The listing builds one solid part. Answer for the finished solid, in the listing's coordinates (mm). A direction names the side the tool comes from. Round coordinates to 2 decimals unless told otherwise and drop trailing zeros. Write each loop counter-clockwise with the first axis right and the second up, starting at its lowest first coordinate (ties: lowest second). Pieces come first, ordered by that corner, then holes.
from build123d import *

# Parameters (mm, degrees)
SKETCH1_W            = 130
SKETCH1_H            = 60
BOSS_EXTRUDE1_DEPTH  = 16
CUT_EXTRUDE1_DEPTH   = 135.372616258
SKETCH3_W            = 18.25
SKETCH3_H            = 5.5
CUT_EXTRUDE2_DEPTH   = 2
BOSS_EXTRUDE2_START  = -2
SKETCH3_7_W          = 0.6
SKETCH3_7_H          = 4.9
SKETCH3_7_H_2        = 3.5
BOSS_EXTRUDE2_DEPTH  = 1
SKETCH3_9_W          = 5.875
SKETCH3_9_H          = 3.5
SKETCH3_9_W_2        = 0.6
SKETCH3_9_H_2        = 4.9
SKETCH3_9_W_3        = 17.05
SKETCH3_9_H_3        = 0.6
BOSS_EXTRUDE3_DEPTH  = 2
SKETCH3_10_W         = 5.875
SKETCH3_10_H         = 3.5
BOSS_EXTRUDE4_DEPTH  = 2
SKETCH4_W            = 25
SKETCH4_H            = 8.5
SKETCH4_H_2          = 6.5
CUT_EXTRUDE3_DEPTH   = 128
BOSS_EXTRUDE10_DEPTH = 100
CHAMFER1_SIZE        = 0.8
CHAMFER2_SIZE        = 2


with BuildPart() as part:
    # Sketch1 → Boss-Extrude1 (new body)
    with BuildSketch(Plane(origin=(0, 0, 0), x_dir=(1, 0, 0), z_dir=(0, 1, 0))):
        Rectangle(SKETCH1_W, SKETCH1_H)
    extrude(amount=BOSS_EXTRUDE1_DEPTH)

    # Sketch2 → Cut-Extrude1 (cut, through all)
    with BuildSketch(Plane(origin=(65, 0, 0), x_dir=(0, 0, -1), z_dir=(1, 0, 0))):
        with BuildLine():
            ThreePointArc((-27.5, 16), (-15, 3.5), (-2.5, 16))
            Line((-2.5, 16), (-27.5, 16))
        make_face()
        with BuildLine():
            Line((-27.5, 16), (-2.5, 16))
            ThreePointArc((-2.5, 16), (-15, 28.5), (-27.5, 16))
        make_face()
    extrude(amount=-CUT_EXTRUDE1_DEPTH, mode=Mode.SUBTRACT)

    # Sketch3 → Cut-Extrude2 (cut)
    with BuildSketch(Plane(origin=(65, 0, 0), x_dir=(0, 0, -1), z_dir=(1, 0, 0))):
        with Locations((15, 13.25)):
            Rectangle(SKETCH3_W, SKETCH3_H)
    extrude(amount=-CUT_EXTRUDE2_DEPTH, mode=Mode.SUBTRACT)

    # Sketch3<7> → Boss-Extrude2 (add)
    with BuildSketch(Plane(origin=(65, 0, 0), x_dir=(0, 0, -1), z_dir=(1, 0, 0)).offset(BOSS_EXTRUDE2_START)):
        with Locations((23.825, 13.55)):
            Rectangle(SKETCH3_7_W, SKETCH3_7_H)
        with Locations((23.825, 17.75)):
            Rectangle(SKETCH3_7_W, SKETCH3_7_H_2)
        with Locations((6.175, 17.75)):
            Rectangle(SKETCH3_7_W, SKETCH3_7_H_2)
        with Locations((6.175, 13.55)):
            Rectangle(SKETCH3_7_W, SKETCH3_7_H)
    extrude(amount=BOSS_EXTRUDE2_DEPTH)

    # Sketch3<9> → Boss-Extrude3 (add)
    with BuildSketch(Plane(origin=(65, 0, 0), x_dir=(0, 0, -1), z_dir=(1, 0, 0))):
        with Locations((2.9375, 17.75)):
            Rectangle(SKETCH3_9_W, SKETCH3_9_H)
        Polygon((0, 0), (30, 0), (30, 16), (24.125, 16), (24.125, 11.1), (24.125, 10.5), (23.525, 10.5), (6.475, 10.5), (5.875, 10.5), (5.875, 11.1), (5.875, 16), (0, 16), align=None)
        with Locations((6.175, 13.55)):
            Rectangle(SKETCH3_9_W_2, SKETCH3_9_H_2)
        with Locations((15, 13.55)):
            Rectangle(SKETCH3_9_W_3, SKETCH3_9_H_2)
        with Locations((6.175, 17.75)):
            Rectangle(SKETCH3_9_W_2, SKETCH3_9_H)
        with Locations((15, 17.75)):
            Rectangle(SKETCH3_9_W_3, SKETCH3_9_H)
        with Locations((15, 10.8)):
            Rectangle(SKETCH3_9_W_3, SKETCH3_9_H_3)
        with Locations((6.175, 10.8)):
            Rectangle(SKETCH3_9_W_2, SKETCH3_9_H_3)
        with Locations((23.825, 13.55)):
            Rectangle(SKETCH3_9_W_2, SKETCH3_9_H_2)
        with Locations((23.825, 10.8)):
            Rectangle(SKETCH3_9_W_2, SKETCH3_9_H_3)
        with Locations((23.825, 17.75)):
            Rectangle(SKETCH3_9_W_2, SKETCH3_9_H)
        with Locations((27.0625, 17.75)):
            Rectangle(SKETCH3_9_W, SKETCH3_9_H)
    extrude(amount=BOSS_EXTRUDE3_DEPTH)

    # Sketch3<10> → Boss-Extrude4 (add)
    with BuildSketch(Plane(origin=(65, 0, 0), x_dir=(0, 0, -1), z_dir=(1, 0, 0))):
        with Locations((2.9375, 17.75)):
            Rectangle(SKETCH3_10_W, SKETCH3_10_H)
        with Locations((27.0625, 17.75)):
            Rectangle(SKETCH3_10_W, SKETCH3_10_H)
    extrude(amount=-BOSS_EXTRUDE4_DEPTH)

    # Sketch4 → Cut-Extrude3 (cut)
    with BuildSketch(Plane.ZY.offset(65)):
        with Locations((-15, 11.75)):
            Rectangle(SKETCH4_W, SKETCH4_H)
        with Locations((-15, 19.25)):
            Rectangle(SKETCH4_W, SKETCH4_H_2)
    extrude(amount=-CUT_EXTRUDE3_DEPTH, mode=Mode.SUBTRACT)

    # Sketch5 → Boss-Extrude10 (add)
    with BuildSketch(Plane.ZY.offset(65)):
        Polygon((1.5, 14), (1.5, 11.5), (-1.5, 11.5), (-1.5, 14), (-5, 14), (-5, 0), (5, 0), (5, 14), align=None)
    extrude(amount=BOSS_EXTRUDE10_DEPTH)

    # Chamfer1
    chamfer1_edges = [part.edges().sort_by_distance(p)[0] for p in [
        (-115, 14, -1.5),
        (-115, 14, 1.5),
    ]]
    chamfer(chamfer1_edges, length=CHAMFER1_SIZE)

    # Chamfer2
    chamfer2_edges = [part.edges().sort_by_distance(p)[0] for p in [
        (-65, 16, -28.75),
        (-65, 16, 28.75),
        (-65, 16, 0),
    ]]
    chamfer(chamfer2_edges, length=CHAMFER2_SIZE - 0.0001)  # a hair under: the kernel refuses the full size


solid = part.part
1. Section A-A on x = -123 is taken. Determine the outline of the cut face in (y, z).
Geometry says:
outline: (0, -5) - (14, -5) - (14, -2.3) - (13.2, -1.5) - (11.5, -1.5) - (11.5, 1.5) - (13.2, 1.5) - (14, 2.3) - (14, 5) - (0, 5) - close
2. Section C-C on x = -43.5 is taken. Determine the outline of the cut face in (y, z), plus the area to 3 significant figures.
Geometry says:
outline: (0, -30) - (16, -30) - (16, -27.5) - (7.5, -27.5) - (7.5, -2.5) - (16, -2.5) - (16, 2.5) arc R12.5 cw to (16, 27.5) - (16, 30) - (0, 30) - close
area: 502 mm2
3. A tool of negligible diameter and unlimited length cuts with its end or side. For faces 4 (the face through (63, 10, -15)), 5 (the face through (-114, 7, -5)), 6 (the face through (65, 3, 15)), 7 (the face through (-2, 12, -27.5)), 8 (the face through (-65, 4, 20)), from which of +Z, -Z, +X, -X, +Y, -Y can it reach the whole face along a straight path? Write none if from no direction.
Geometry says:
face 4: +Y
face 5: -Z, -X, +Y, -Y
face 6: +Z, +X, +Y, -Y
face 7: -X, +Y
face 8: +Z, -X, +Y, -Y
4. Given pin 1 (7 mm diameter, centred on y = 5, z = -21, fed in from -X); pin 2 (11 mm diameter, centred on x = -133, y = 8, fed in from +Z); pin 3 (3 mm diameter, centred on x = -13, z = 29, fed in from +Y), each flat-ended and moving along its own axis, determine where each tip first touches the part or whether it passes through.
Geometry says:
pin 1: stops at x = -65
pin 2: stops at z = 5
pin 3: stops at y = 16
5. Section B-B on z = 15 is taken. Determine the outline of the cut face in (x, y), plus the area to 3 significant figures.
Geometry says:
outline: (-65, 0) - (65, 0) - (65, 3.5) - (-65, 3.5) - close
area: 455 mm2
6. For a pull along X with two mould halves and no side action, classify faces 1 (the face through (0.91, 3.503, 15.275)), 2 (the face through (-65, 4, -17)), 3 (the face through (-2, 12, -2.5)) as released by +X, released by -X, zero draft, split by the parting line, or undercut.
Geometry says:
face 1: zero draft
face 2: released by -X
face 3: undercut
7. Straight lines are drawn through the part: line 1 along Z through (x, y) = (1, 12); line 2 along Z through (x, y) = (-55, 11.5); line 3 along X through (y, z) = (3.75, -7). For each, find the intervals that lie inside material, in ascending order.
Geometry says:
line 1: z = -30 to -27.5, -2.5 to 3.16, 26.84 to 30
line 2: z = -30 to -27.5, -2.5 to 3.34, 26.66 to 30
line 3: x = -65 to 67
